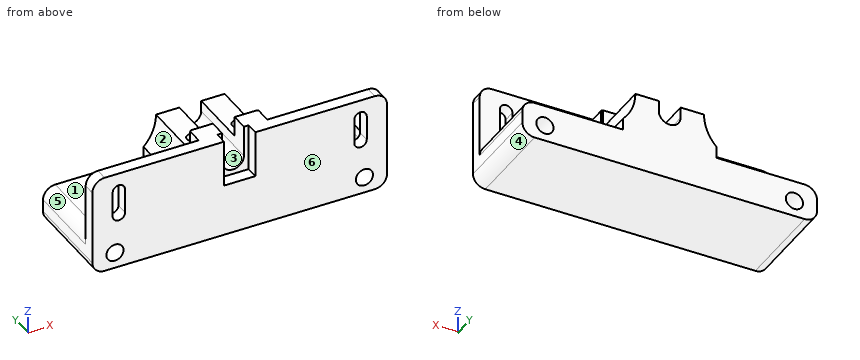
```python
from build123d import *

# Parameters (mm, degrees)
SKETCH1_W                  = 38.1
SKETCH1_H                  = 25.4
BOSS_EXTRUDE1_DEPTH        = 25.0825
CUT_EXTRUDE3_DEPTH         = 26.4
CUT_EXTRUDE4_DEPTH         = 26.4
CUT_EXTRUDE5_DEPTH         = 26.4
BOSS_EXTRUDE2_DEPTH        = 6.985
BOSS_EXTRUDE3_DEPTH        = 5.08
SKETCH29_W                 = 19.05
SKETCH29_H                 = 5.08
CUT_EXTRUDE6_DEPTH         = 1.905
SKETCH30_W                 = 19.05
SKETCH30_H                 = 5.08
CUT_EXTRUDE7_DEPTH         = 1.905
CUT_EXTRUDE10_REACH        = 39.465
CUT_EXTRUDE11_REACH        = 39.465
SKETCH77_W                 = 1.4732
SKETCH77_H                 = 16.0274
M2_5_CLEARANCE_HOLE1_D     = 2.9464
M2_5_CLEARANCE_HOLE1_DEPTH = 25.0825
CHAMFER1_SIZE              = 0.511100582
CHAMFER1_SIZE2             = 0.522104304
CHAMFER2_SIZE              = 0.558247665
CHAMFER2_SIZE2             = 0.538663646
SKETCH80_W                 = 38.1
SKETCH80_H                 = 25.4
CUT_EXTRUDE13_DEPTH        = 7.9375
SKETCH81_W                 = 120
SKETCH81_H                 = 15
BOSS_EXTRUDE4_DEPTH        = 37.465
SKETCH82_R                 = 3.5
CUT_EXTRUDE14_DEPTH        = 38.465
FILLET3_R                  = 5
FILLET4_R                  = 5
FILLET5_R                  = 5
SKETCH83_R                 = 2.4003
CUT_EXTRUDE15_DEPTH        = 7.1374


with BuildPart() as part:
    # Sketch1 → Boss-Extrude1 (new body)
    with BuildSketch(Plane(origin=(0, 0, -20.6375), x_dir=(-1, 0, 0), z_dir=(0, 0, -1))):
        with Locations((0, 12.7)):
            Rectangle(SKETCH1_W, SKETCH1_H)
    extrude(amount=-BOSS_EXTRUDE1_DEPTH)

    # Sketch18 → Cut-Extrude3 (cut, through all)
    with BuildSketch(Plane(origin=(0, 0, 0), x_dir=(-1, 0, 0), z_dir=(0, -1, 0))):
        with BuildLine():
            Line((13.97, -4.445), (19.05, -4.445))
            Line((19.05, -4.445), (19.05, 7.9375))
            ThreePointArc((19.05, 7.9375), (15.289364951, 2.247023353), (13.97, -4.445))
        make_face()
    extrude(amount=-CUT_EXTRUDE3_DEPTH, mode=Mode.SUBTRACT)

    # Sketch19 → Cut-Extrude4 (cut, through all)
    with BuildSketch(Plane.XZ):
        with BuildLine():
            Line((4.445, 4.445), (-4.445, 4.445))
            Line((-4.445, 4.445), (-4.445, 0))
            ThreePointArc((-4.445, 0), (0, -4.445), (4.445, 0))
            Line((4.445, 0), (4.445, 4.445))
        make_face()
    extrude(amount=-CUT_EXTRUDE4_DEPTH, mode=Mode.SUBTRACT)

    # Sketch20 → Cut-Extrude5 (cut, through all)
    with BuildSketch(Plane.XZ):
        with BuildLine():
            Line((19.05, -7.9375), (19.05, 4.445))
            Line((19.05, 4.445), (13.97, 4.445))
            ThreePointArc((13.97, 4.445), (15.289364951, -2.247023353), (19.05, -7.9375))
        make_face()
    extrude(amount=-CUT_EXTRUDE5_DEPTH, mode=Mode.SUBTRACT)

    # Sketch21 → Boss-Extrude2 (add)
    with BuildSketch(Plane.XZ):
        with BuildLine():
            Line((4.445, 0), (4.445, 12.7))
            Line((4.445, 12.7), (13.97, 12.7))
            Line((13.97, 12.7), (13.97, 4.445))
            ThreePointArc((13.97, 4.445), (15.289364951, -2.247023353), (19.05, -7.9375))
            Line((19.05, -7.9375), (-19.05, -7.9375))
            ThreePointArc((-19.05, -7.9375), (-15.289364951, -2.247023353), (-13.97, 4.445))
            Line((-13.97, 4.445), (-13.97, 12.7))
            Line((-13.97, 12.7), (-4.445, 12.7))
            Line((-4.445, 12.7), (-4.445, 0))
            ThreePointArc((-4.445, 0), (0, -4.445), (4.445, 0))
        make_face()
    extrude(amount=BOSS_EXTRUDE2_DEPTH)

    # Sketch22 → Boss-Extrude3 (add)
    with BuildSketch(Plane.XZ.offset(6.985)):
        Polygon((-4.445, -6.35), (4.445, -6.35), (4.445, 12.7), (60, 12.7), (60, -12.7), (-60, -12.7), (-60, 12.7), (-4.445, 12.7), align=None)
    extrude(amount=BOSS_EXTRUDE3_DEPTH)

    # Sketch29 → Cut-Extrude6 (cut)
    with BuildSketch(Plane.ZY.offset(-4.445)):
        with Locations((3.175, -9.525)):
            Rectangle(SKETCH29_W, SKETCH29_H)
    extrude(amount=-CUT_EXTRUDE6_DEPTH, mode=Mode.SUBTRACT)

    # Sketch30 → Cut-Extrude7 (cut)
    with BuildSketch(Plane(origin=(-4.445, 0, 0), x_dir=(0, 0, -1), z_dir=(1, 0, 0))):
        with Locations((-3.175, -9.525)):
            Rectangle(SKETCH30_W, SKETCH30_H)
    extrude(amount=-CUT_EXTRUDE7_DEPTH, mode=Mode.SUBTRACT)

    # Sketch48 → Cut-Extrude10 (cut, up to next)
    with BuildSketch(Plane(origin=(0, -12.065, 0), x_dir=(-1, 0, 0), z_dir=(0, -1, 0)), mode=Mode.PRIVATE) as cut_extrude10_sk1:
        with BuildLine():
            Line((-51.7525, 5.08), (-51.7525, -5.08))
            ThreePointArc((-51.7525, -5.08), (-49.2125, -7.62), (-46.6725, -5.08))
            Line((-46.6725, -5.08), (-46.6725, 5.08))
            ThreePointArc((-46.6725, 5.08), (-49.2125, 7.62), (-51.7525, 5.08))
        make_face()
    cut_extrude10_tool1 = extrude(cut_extrude10_sk1.sketch, amount=-CUT_EXTRUDE10_REACH, mode=Mode.PRIVATE) & part.part
    add(cut_extrude10_tool1.solids().sort_by_distance((49.2125, -12.065, 0))[0], mode=Mode.SUBTRACT)

    # Sketch57 → Cut-Extrude11 (cut, up to next)
    with BuildSketch(Plane(origin=(0, -12.065, 0), x_dir=(-1, 0, 0), z_dir=(0, -1, 0)), mode=Mode.PRIVATE) as cut_extrude11_sk1:
        with BuildLine():
            Line((46.6725, 5.08), (46.6725, -5.08))
            ThreePointArc((46.6725, -5.08), (49.2125, -7.62), (51.7525, -5.08))
            Line((51.7525, -5.08), (51.7525, 5.08))
            ThreePointArc((51.7525, 5.08), (49.2125, 7.62), (46.6725, 5.08))
        make_face()
    cut_extrude11_tool1 = extrude(cut_extrude11_sk1.sketch, amount=-CUT_EXTRUDE11_REACH, mode=Mode.PRIVATE) & part.part
    add(cut_extrude11_tool1.solids().sort_by_distance((-49.2125, -12.065, 0))[0], mode=Mode.SUBTRACT)

    # Sketch77 → Cut-Revolve2 (revolve, cut)
    with BuildSketch(Plane(origin=(0, 6.35, 0), x_dir=(1, 0, 0), z_dir=(0, 1, 0))):
        with Locations((9.9441, 12.6238)):
            Rectangle(SKETCH77_W, SKETCH77_H)
    revolve(axis=Axis((9.2075, 6.35, -20.6375), (0, 0, 1)), mode=Mode.SUBTRACT)

    # M2.5 Clearance Hole1
    with Locations(Plane.XY.offset(4.445)):
        with Locations((9.2075, 6.35), (-9.2075, 6.35)):
            Hole(M2_5_CLEARANCE_HOLE1_D / 2, depth=M2_5_CLEARANCE_HOLE1_DEPTH)

    # Chamfer1
    chamfer1_edges = [part.edges().sort_by_distance(p)[0] for p in [
        (13.97, 0, 8.5725),
    ]]
    chamfer1_side = [part.faces().sort_by_distance(p)[0] for p in [
        (13.97, -3.4925, 8.5725),
    ]]
    chamfer(chamfer1_edges, length=CHAMFER1_SIZE, length2=CHAMFER1_SIZE2, reference=chamfer1_side[0])

    # Chamfer2
    chamfer2_edges = [part.edges().sort_by_distance(p)[0] for p in [
        (-13.97, 0, 8.5725),
    ]]
    chamfer2_side = [part.faces().sort_by_distance(p)[0] for p in [
        (-13.97, -3.4925, 8.5725),
    ]]
    chamfer(chamfer2_edges, length=CHAMFER2_SIZE, length2=CHAMFER2_SIZE2, reference=chamfer2_side[0])

    # Sketch80 → Cut-Extrude13 (cut)
    with BuildSketch(Plane(origin=(0, 0, -20.6375), x_dir=(-1, 0, 0), z_dir=(0, 0, -1))):
        with Locations((0, 12.7)):
            Rectangle(SKETCH80_W, SKETCH80_H)
    extrude(amount=-CUT_EXTRUDE13_DEPTH, mode=Mode.SUBTRACT)

    # Sketch81 → Boss-Extrude4 (add)
    with BuildSketch(Plane(origin=(0, 25.4, 0), x_dir=(1, 0, 0), z_dir=(0, 1, 0))):
        with Locations((0, 20.2)):
            Rectangle(SKETCH81_W, SKETCH81_H)
    extrude(amount=-BOSS_EXTRUDE4_DEPTH)

    # Sketch82 → Cut-Extrude14 (cut, through all)
    with BuildSketch(Plane.XZ.offset(12.065)):
        with Locations((-50.8, -21.156433146)):
            Circle(SKETCH82_R)
        with Locations((50.8, -21.156433146)):
            Circle(SKETCH82_R)
    extrude(amount=-CUT_EXTRUDE14_DEPTH, mode=Mode.SUBTRACT)

    # Fillet3
    fillet3_edges = [part.edges().sort_by_distance(p)[0] for p in [
        (60, 6.6675, -27.7),
        (-60, 6.6675, -27.7),
    ]]
    fillet(fillet3_edges, radius=FILLET3_R)

    # Fillet4
    fillet4_edges = [part.edges().sort_by_distance(p)[0] for p in [
        (60, 9.2075, -12.7),
        (-60, 9.2075, -12.7),
    ]]
    fillet(fillet4_edges, radius=FILLET4_R)

    # Fillet5
    fillet5_edges = [part.edges().sort_by_distance(p)[0] for p in [
        (-60, -9.525, 12.7),
        (60, -9.525, 12.7),
    ]]
    fillet(fillet5_edges, radius=FILLET5_R)

    # Sketch83 → Cut-Extrude15 (cut)
    with BuildSketch(Plane.XY.offset(4.445)):
        with Locations((-9.2075, 6.35)):
            Circle(SKETCH83_R)
        with Locations((9.2075, 6.35)):
            Circle(SKETCH83_R)
    extrude(amount=-CUT_EXTRUDE15_DEPTH, mode=Mode.SUBTRACT)


solid = part.part
```
Could you check a few things on this model? Use its own coordinates, in mm. Face numbers are marked on the shaded views. A direction names the side the tool comes from. Coordinates: 2 decimals unless noted, no trailing zeros. Loops run counter-clockwise (first coordinate to the right, second up) from the corner with the lowest first, then second, coordinate; pieces in that order, holes last. Notation, with made-up numbers: M 38,-17 L 88,-17 A19 cw 88,15 Z; hole C 10,-28 d9. An arc over 180 degrees is marked long. Put each result on its own line as item: value. Start each with the question number.
(1) I need wall thicknesses on line 1 (X direction, y = 14.5, z = -21.5); line 2 (Y direction, x = 1, z = -11) (3 decimals); line 3 (Z direction, x = 50.8, y = 16.5). Which ranges of each line are inside material? Lowest first, please. Write a range as from..to.
(2) Thinking about a two-plate mould opening in X: for the marked faces 1, 2, 3 and 4, which applies, pulls with the +X half, pulls with the -X half, needs draft (parallel to the pull), parting line crosses it, or undercut?
(3) Suppose I cut it at D-D on x = 45. Please give me the cut outline in (y, z) (3 decimals).
(4) Suppose I cut it at A-A on z = -10. Count the separate pieces of the cut face and the enclosed holes in it, then the cut area to 3 significant figures.
(5) Will these pins go through, and if not, where does the flat tip stop? P1, Ø3, axis at x = -9.5, y = 6, coming from the +Z side; P2, Ø3, axis at y = -5, z = 10, coming from the +X side; P3, Ø1, axis at x = -44.5, z = 3.5, coming from the +Y side (3 decimals).
(6) For the marked faces 5 and 6, which set-ups out of +Z, -Z, +X, -X, +Y, -Y let a thin tool reach every point of the face, with its end or its side?
Solutions:
1. line 1: x = -60..-54.28, -47.32..47.32, 54.28..60
1. line 2: y = -12.065..-6.985, 0..25.4
1. line 3: z = -27.7..-24.66, -17.66..-12.7
2. face 1: needs draft
2. face 2: pulls with the -X half
2. face 3: undercut
2. face 4: pulls with the +X half
3. outline: M -12.065,-27.7 L 25.4,-27.7 L 25.4,-12.7 L -6.985,-12.7 L -6.985,12.7 L -12.065,12.7 Z
4. separate pieces: 2
4. enclosed holes: 2
4. area: 1,560 mm2
5. P1: stops at z = -2.69
5. P2: stops at x = 13.97
5. P3: stops at y = -6.985
6. face 5: +Z, -X, +Y
6. face 6: +Z, -Z, +X, -X, -Y
